Study the drawing (mm; zero at the part's minimum x, y, z) and answer. Coordinates: 2 decimals unless noted, no trailing zeros. Loops run counter-clockwise (first coordinate to the right, second up) from the corner with the lowest first, then second, coordinate; pieces in that order, holes last. Notation, with made-up numbers: (63.5, -33.75) -> (120.5, -33.75) arc R12 cw to (120.5, -20.75) -> close; hole circle Ø1 at (35.25, -29). An arc over 180 degrees is marked (long way). Answer as CSV lines item,"result".
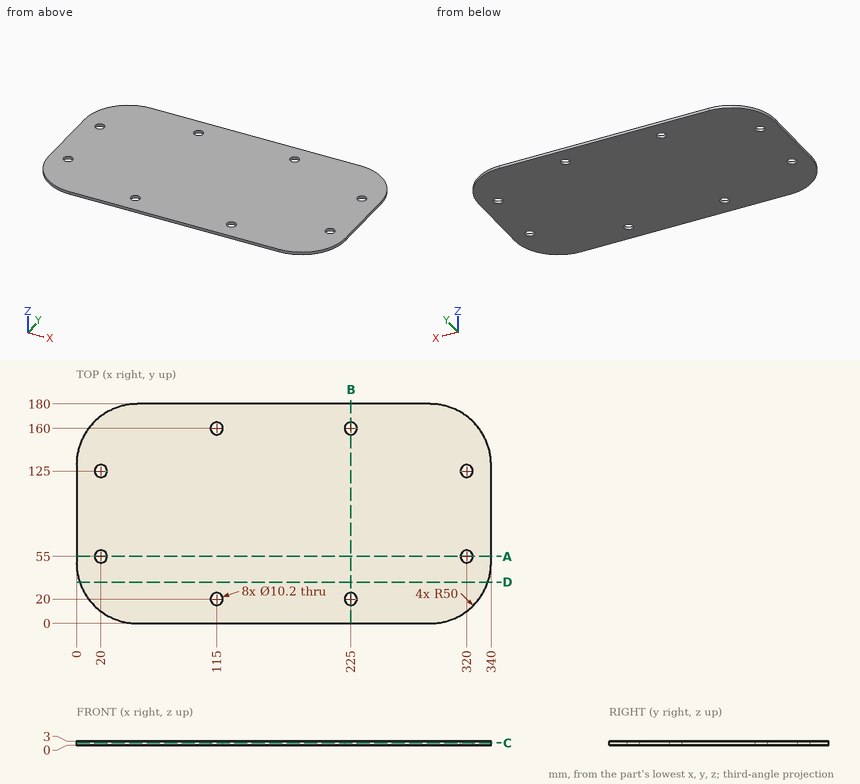
Q1. A cutting plane is placed at A-A, the plane y = 55. Write down the section's boundary in (x, z).
Results:
outline,"(0, 0) -> (14.9, 0) -> (14.9, 3) -> (0, 3) -> close; (25.1, 0) -> (314.9, 0) -> (314.9, 3) -> (25.1, 3) -> close; (325.1, 0) -> (340, 0) -> (340, 3) -> (325.1, 3) -> close"
Q2. Given pin 1 Ø9 at (x, y) = (20, 125) entering from +Z, flat-ended and moving along its own axis, determine where the tip first touches the part or whether it passes through.
Results:
pin 1,"passes through"
Q3. A cutting plane is placed at C-C, the plane z = 1.9. Give the number of separate pieces and of enclosed holes in the cut face, and give its area (3 significant figures).
Results:
separate pieces,"1"
enclosed holes,"8"
area,"58,400 mm²"
Q4. Find the intervals of material crossed by probe 1 along Y at (x, z) = (225, 1.8); probe 2 along Y at (x, z) = (111.5, 2.5); probe 3 along X at (y, z) = (164, 2.7), in increasing order. Write a range as [from, to].
Results:
probe 1,"y = [0, 14.9], [25.1, 154.9], [165.1, 180]"
probe 2,"y = [0, 16.29], [23.71, 156.29], [163.71, 180]"
probe 3,"x = [13.34, 111.84], [118.16, 221.84], [228.16, 326.66]"
Q5. A cutting plane is placed at D-D, the plane y = 34. Write down the section's boundary in (x, z).
Results:
outline,"(2.63, 0) -> (337.37, 0) -> (337.37, 3) -> (2.63, 3) -> close"
Q6. A cutting plane is placed at B-B, the plane x = 225. Write down the section's boundary in (y, z).
Results:
outline,"(0, 0) -> (14.9, 0) -> (14.9, 3) -> (0, 3) -> close; (25.1, 0) -> (154.9, 0) -> (154.9, 3) -> (25.1, 3) -> close; (165.1, 0) -> (180, 0) -> (180, 3) -> (165.1, 3) -> close"
